from build123d import *

# Parameters (mm, degrees)
F1_DEPTH = 100


with BuildPart() as f1:
    # F0 (on Top) → F1 (new body)
    with BuildSketch(Plane.XY):
        Polygon((513.63961, 63.63961), (450, 0), (450, -25), (467.320508, -35), (467.320508, -55), (450, -65), (450, -85.550674), (479.830233, -102.38872), (480.166933, -137.0281), (450.336699, -154.63938), (450, -154.449326), (450, -179.204377), (489.648216, -201.307126), (490.342739, -247.489925), (450.694523, -271.1828), (450, -270.795623), (450, -302.53674), (450.476343, -302.266938), (500.23647, -331.545994), (499.760127, -389.279056), (450, -417.46326), (450, -450), (513.63961, -513.63961), align=None)
        Polygon((467.320508, -35), (450, -25), (450, -65), (467.320508, -55), align=None)
        Polygon((450, -65), (450, -25), (432.679492, -35), (432.679492, -55), align=None)
        Polygon((450, -154.449326), (450, -85.550674), (449.663301, -85.36062), (419.833067, -102.9719), (420.169767, -137.61128), align=None)
        Polygon((479.830233, -102.38872), (450, -85.550674), (450, -154.449326), (450.336699, -154.63938), (480.166933, -137.0281), align=None)
        Polygon((489.648216, -201.307126), (450, -179.204377), (450, -270.795623), (450.694523, -271.1828), (490.342739, -247.489925), align=None)
        Polygon((450, -270.795623), (450, -179.204377), (449.305477, -178.8172), (409.657261, -202.510075), (410.351784, -248.692874), align=None)
        Polygon((449.523657, -417.733062), (450, -417.46326), (450, -302.53674), (400.239873, -330.720944), (399.76353, -388.454006), align=None)
        Polygon((450, -302.53674), (450, -417.46326), (499.760127, -389.279056), (500.23647, -331.545994), (450.476343, -302.266938), align=None)
    extrude(amount=F1_DEPTH)


solid = f1.part
Model file for the job. Use its own axes, mm. A direction names the side the tool comes from. Round coordinates to 2 decimals unless told otherwise and drop trailing zeros. Order: outer loops, then holes, each group sorted by start corner. A loop starts at its lowest first (then second) coordinate and runs counter-clockwise, first axis right, second up. Notation, with made-up numbers: M 1.25,85 L 38.25,85 A17 cw 38.25,91 Z; hole C -27.5,76.25 d10. An arc over 180 degrees is marked long. Write each question's results on one line, items separated by ' | '. Start each with the question number.
(1) Saw through at B-B, the plane z = 21.5. Give the cut face in (x, y), then the cut area to 3 significant figures.
(2) Which spindle directions (+Z, -Z, +X, -X, +Y, -Y) get a long thin tool onto all of the face, cutting with end or side? Do faces 1 (the face through (450, -75, 49)), 2 (the face through (469, -221, 0)), 3 (the face through (450, -12, 49)), 4 (the face through (469, -221, 100)), 5 (the face through (450, -434, 49)). Say none if no direction does.
(3) Saw through at A-A, the plane x = 442. Give the cut face in (y, z).
(4) Probe probe 1 along Y at (x, z) = (425, 86); probe 2 along Y at (x, z) = (433, 61); probe 3 along Y at (x, z) = (430, 79). List the from-to ranges inside material, lowest first. Write a range as from..to.
(5) Saw through at C-C, the plane y = 26.5. Give the cut face in (x, z), then the cut area to 3 significant figures.
(6) Drop flat-ended pins along their axis: pin 1 (5 mm diameter, centred on y = -216.5, z = 84, fed in from -X); pin 2 (5 mm diameter, centred on x = 495.5, z = 12, fed in from +Y); pin 3 (10 mm diameter, centred on y = -172.5, z = 48.5, fed in from -X). Give the stop position or say it passes through.
(7) Saw through at D-D, the plane x = 499.5. Give the cut face in (y, z), then the cut area to 3 significant figures.
(8) Two-plate mould, pull along Y, no slides. Class faces 6 (the face through (434.876, -145.912, 49.3)), 7 (the face through (482, 32, 49)), 8 (the face through (424.3, -402.89, 49.3)): pulls with the +Y half, pulls with the -Y half, needs draft (parallel to the pull), parting line crosses it, or undercut.
Established:
1) outline: M 399.76,-388.45 L 449.52,-417.73 L 450,-417.46 L 450,-450 L 513.64,-513.64 L 513.64,63.64 L 450,0 L 450,-25 L 432.68,-35 L 432.68,-55 L 450,-65 L 450,-85.55 L 449.66,-85.36 L 419.83,-102.97 L 420.17,-137.61 L 450,-154.45 L 450,-179.2 L 449.31,-178.82 L 409.66,-202.51 L 410.35,-248.69 L 450,-270.8 L 450,-302.54 L 400.24,-330.72 Z | area: 41,900 mm^2
2) face 1: +Z, -Z, -X | face 2: -Z, +X, -X, +Y, -Y | face 3: +Z, -Z, -X, +Y | face 4: +Z, +X, -X, +Y, -Y | face 5: +Z, -Z, -X, -Y
3) outline: M -413.31,0 L -307.07,0 L -307.07,100 L -413.31,100 Z; M -266.34,0 L -183.18,0 L -183.18,100 L -266.34,100 Z; M -149.93,0 L -89.88,0 L -89.88,100 L -149.93,100 Z; M -60.38,0 L -29.62,0 L -29.62,100 L -60.38,100 Z
4) probe 1: y = -403.3..-316.7, -256.86..-193.34, -140.34..-99.92 | probe 2: y = -408.01..-312.17, -261.32..-188.56, -144.85..-95.2, -55.19..-34.81 | probe 3: y = -406.25..-313.86, -259.65..-190.35, -143.16..-96.97
5) outline: M 476.5,0 L 513.64,0 L 513.64,100 L 476.5,100 Z | area: 3,710 mm^2
6) pin 1: stops at x = 409.83 | pin 2: stops at y = 48 | pin 3: stops at x = 450
7) outline: M -499.5,0 L 49.5,0 L 49.5,100 L -499.5,100 Z | area: 54,900 mm^2
8) face 6: undercut | face 7: pulls with the +Y half | face 8: pulls with the -Y half
